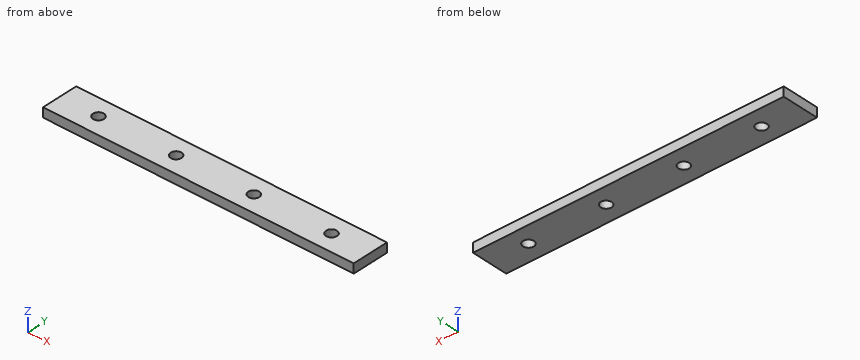
```python
from build123d import *

# Parameters (mm, degrees)
SKETCH1_W           = 100
SKETCH1_H           = 12
BOSS_EXTRUDE1_DEPTH = 3
SKETCH7_R           = 1.75
CUT_EXTRUDE1_DEPTH  = 4
LPATTERN1_COUNT     = 4
LPATTERN1_PITCH     = 25


with BuildPart() as part:
    # Sketch1 → Boss-Extrude1 (new body)
    with BuildSketch(Plane.XY):
        Rectangle(SKETCH1_W, SKETCH1_H)
    extrude(amount=BOSS_EXTRUDE1_DEPTH)

    # Sketch7 → Cut-Extrude1 (cut, through all)
    with BuildSketch(Plane.XY.offset(3)):
        with Locations((37.5, 0)):
            Circle(SKETCH7_R)
    cut_extrude1 = extrude(amount=-CUT_EXTRUDE1_DEPTH, mode=Mode.SUBTRACT)

    # LPattern1: Cut-Extrude1 ×4
    with Locations(*[(-i * LPATTERN1_PITCH, 0, 0) for i in range(1, LPATTERN1_COUNT)]):
        add(cut_extrude1, mode=Mode.SUBTRACT)


solid = part.part
```
Read the model definition and answer for the solid it produces. Units are mm, in the model's axes. Coordinates: 2 decimals unless noted, no trailing zeros. Write each loop counter-clockwise with the first axis right and the second up, starting at its lowest first coordinate (ties: lowest second). Pieces come first, ordered by that corner, then holes. Notation, with made-up numbers: (-31.75, -20.75) -> (27.25, -20.75) arc R23 ccw to (27.25, 18.25) -> close; hole circle Ø11 at (38.5, 62.25). An arc over 180 degrees is marked (long way). Answer as a JSON object with one key per item and string values.
Q1. The part is cut by section B-B on x = -37.5. Give the vertices of the cut face in (y, z).
The answers:
{"outline": "(-6, 0) -> (-1.75, 0) -> (-1.75, 3) -> (-6, 3) -> close; (1.75, 0) -> (6, 0) -> (6, 3) -> (1.75, 3) -> close"}
Q2. Flat-ended cylindrical pins translate along their axes: pin 1 Ø4.5 at (x, y) = (37.5, 0) entering from -Z; pin 2 Ø3 at (x, y) = (-12.5, 0) entering from +Z. Find the tip coordinate at first contact, or state that the pin passes through.
The answers:
{"pin 1": "stops at z = 0", "pin 2": "passes through"}
Q3. The part is cut by section A-A on z = 2.4. Give the vertices of the cut face in (x, y), then the cut area to 3 significant figures.
The answers:
{"outline": "(-50, -6) -> (50, -6) -> (50, 6) -> (-50, 6) -> close; hole circle Ø3.5 at (-37.5, 0); hole circle Ø3.5 at (-12.5, 0); hole circle Ø3.5 at (12.5, 0); hole circle Ø3.5 at (37.5, 0)", "area": "1,160 mm2"}
Q4. The part is cut by section C-C on y = 0. Give the vertices of the cut face in (x, z), then the cut area to 3 significant figures.
The answers:
{"outline": "(-50, 0) -> (-39.25, 0) -> (-39.25, 3) -> (-50, 3) -> close; (-35.75, 0) -> (-14.25, 0) -> (-14.25, 3) -> (-35.75, 3) -> close; (-10.75, 0) -> (10.75, 0) -> (10.75, 3) -> (-10.75, 3) -> close; (14.25, 0) -> (35.75, 0) -> (35.75, 3) -> (14.25, 3) -> close; (39.25, 0) -> (50, 0) -> (50, 3) -> (39.25, 3) -> close", "area": "258 mm2"}
Q5. Consider line 1 (X direction, y = 0.5, z = 0.1); line 2 (Y direction, x = 12.5, z = 0.7). Determine where each line is inside the solid, lowest interval first. Write a range as [from, to].
The answers:
{"line 1": "x = [-50, -39.18], [-35.82, -14.18], [-10.82, 10.82], [14.18, 35.82], [39.18, 50]", "line 2": "y = [-6, -1.75], [1.75, 6]"}
